Verification items for this drawing (mm, ordinates from the low corner). A direction names the side the tool comes from. Round coordinates to 2 decimals unless told otherwise and drop trailing zeros. Write each loop counter-clockwise with the first axis right and the second up, starting at its lowest first coordinate (ties: lowest second). Pieces come first, ordered by that corner, then holes. Notation, with made-up numbers: (-4.5, -33.5) -> (12.5, -33.5) arc R28 ccw to (12.5, 3.5) -> close; hole circle Ø11 at (1.5, 6). An arc over 180 degrees is marked (long way). Use one line per item in the form item = value. Start each with the question number.
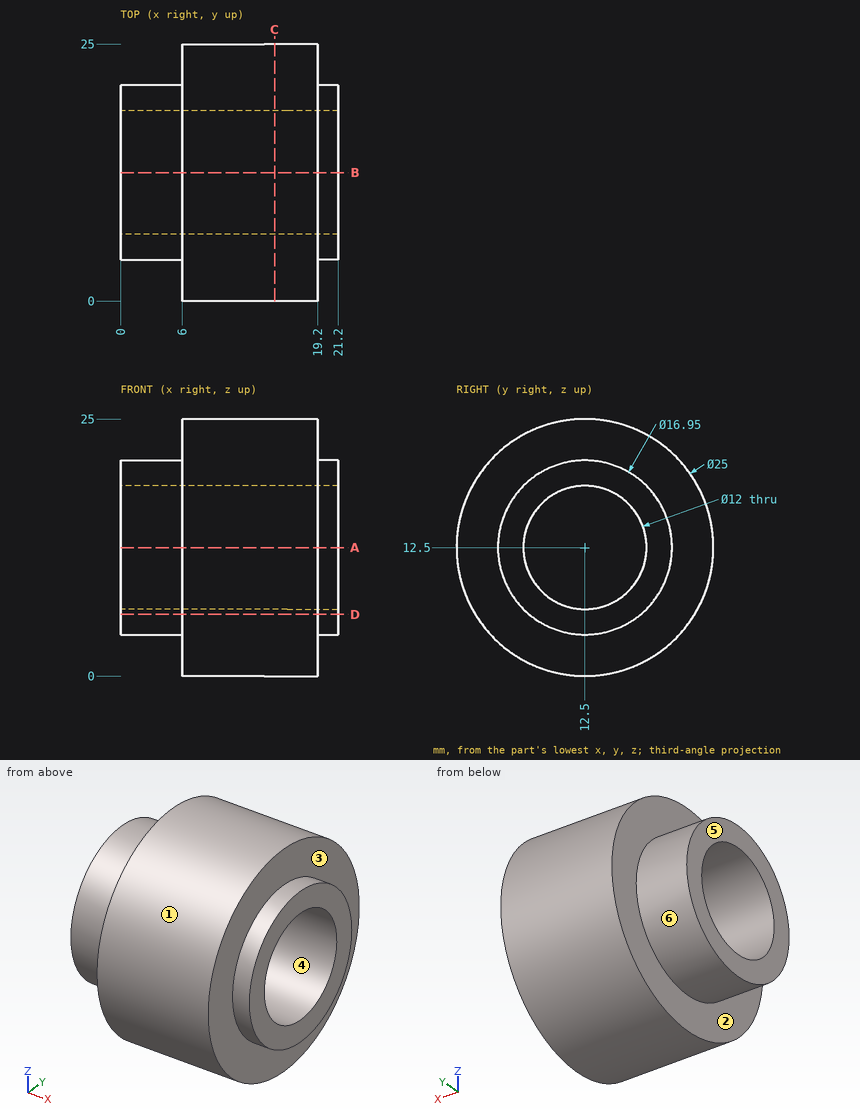
1. Mould release check, pull along Y, two halves, no side actions. Record for the marked faces 4, 5 and 6: +Y half, -Y half, draft (parallel to the pull), parting line (faces both ways), or undercut.
2. Scan lines: probe 1 along Z at (x, y) = (6.5, 12.5); probe 2 along X at (y, z) = (5.25, 5). Record each from-to range of solid material in increasing order.
3. Tool access check on the marked faces 1, 2 and 3. Record the directions out of +Z, -Z, +X, -X, +Y, -Y that give a thin tool (end or side, any length) a straight path to the whole face; none if there is none.
4. Depth check by flat-ended pin: pin 1 (12 mm diameter, centred on x = 14.5, y = 19, fed in from -Z); pin 2 (1.5 mm diameter, centred on x = 5.5, y = 14, fed in from +Z); pin 3 (8 mm diameter, centred on y = 15.5, z = 7.5, fed in from -X); pin 4 (2 mm diameter, centred on x = 3.5, y = 19, fed in from +Z). Enter the tip coordinate at first touch or a pass-through.
5. Sectioned sample at A-A (z = 12.5). Enter the section's corners in (x, y) (3 decimals), and give its area (3 significant figures).
6. Sectioned sample at C-C (x = 15). Enter the section's corners in (y, z).
7. Sectioned sample at D-D (z = 6). Enter the section's corners in (x, y).
Returned:
q1.face_4 = undercut
q1.face_5 = draft
q1.face_6 = parting line
q2.probe_1 = 0 to 6.5, 18.5 to 25
q2.probe_2 = 6 to 19.2
q3.face_1 = +X, -X
q3.face_2 = -X
q3.face_3 = +X
q4.pin_1 = 0.01
q4.pin_2 = 24.96
q4.pin_3 = 0
q4.pin_4 = 18.95
q5.outline = (0, 4.025) -> (6, 4.025) -> (6, 0) -> (19.2, 0) -> (19.2, 4.025) -> (21.2, 4.025) -> (21.2, 6.5) -> (0, 6.5) -> close; (0, 18.5) -> (21.2, 18.5) -> (21.2, 20.975) -> (19.2, 20.975) -> (19.2, 25) -> (6, 25) -> (6, 20.975) -> (0, 20.975) -> close
q5.area = 211 mm^2
q6.outline = circle Ø25 at (12.5, 12.5); hole circle Ø12 at (12.5, 12.5)
q7.outline = (0, 7.06) -> (6, 7.06) -> (6, 1.82) -> (19.2, 1.82) -> (19.2, 7.06) -> (21.2, 7.06) -> (21.2, 17.94) -> (19.2, 17.94) -> (19.2, 23.18) -> (6, 23.18) -> (6, 17.94) -> (0, 17.94) -> close
